from build123d import *

# Parameters (mm, degrees)
SKETCH_1_R          = 17.2
EXTRUDE_1_DEPTH     = 45
SKETCH_2_R          = 18.5
EXTRUDE_2_DEPTH     = 27
SKETCH_6_R          = 1.5
CUT_EXTRUDE_1_DEPTH = 10
SKETCH_3_R          = 6
EXTRUDE_3_DEPTH     = 8
SKETCH_4_R          = 3
EXTRUDE_4_DEPTH     = 15.5


with BuildPart() as part:
    # 草图1 → 凸台-拉伸1 (new body)
    with BuildSketch(Plane.XY):
        with Locations(Location((0, 0, 0), (0, 0, 180))):
            Circle(SKETCH_1_R)
    extrude(amount=EXTRUDE_1_DEPTH)

    # 草图2 → 凸台-拉伸2 (add)
    with BuildSketch(Plane.XY.offset(45)):
        Circle(SKETCH_2_R)
    extrude(amount=EXTRUDE_2_DEPTH)

    # 草图6 → 切除-拉伸1 (cut)
    with BuildSketch(Plane.XY.offset(72)):
        with Locations((-15.5, 0)):
            Circle(SKETCH_6_R)
        with Locations((-7.75, 13.423393759)):
            Circle(SKETCH_6_R)
        with Locations((7.75, 13.423393759)):
            Circle(SKETCH_6_R)
        with Locations((15.5, 0)):
            Circle(SKETCH_6_R)
        with Locations((7.75, -13.423393759)):
            Circle(SKETCH_6_R)
        with Locations((-7.75, -13.423393759)):
            Circle(SKETCH_6_R)
    extrude(amount=-CUT_EXTRUDE_1_DEPTH, mode=Mode.SUBTRACT)

    # 草图3 → 凸台-拉伸3 (add)
    with BuildSketch(Plane.XY.offset(72)):
        with Locations((0, 7)):
            Circle(SKETCH_3_R)
    extrude(amount=EXTRUDE_3_DEPTH)

    # 草图4 → 凸台-拉伸4 (add)
    with BuildSketch(Plane.XY.offset(80)):
        with Locations((0, 7)):
            Circle(SKETCH_4_R)
    extrude(amount=EXTRUDE_4_DEPTH)


solid = part.part
Part model, mm, in its own coordinate system. A direction names the side the tool comes from. Coordinates: 2 decimals unless noted, no trailing zeros. Loops run counter-clockwise (first coordinate to the right, second up) from the corner with the lowest first, then second, coordinate; pieces in that order, holes last. Notation, with made-up numbers: (39, -2.5) -> (56, -2.5) arc R12 cw to (56, 15.5) -> close; hole circle Ø9 at (4.5, 57.5). An arc over 180 degrees is marked (long way). Use a Markdown table: item, result. Add a question column.
Item 1: Probe probe 1 along Y at (x, z) = (-7.75, 67.25); probe 2 along Y at (x, z) = (7, 68); probe 3 along Z at (x, y) = (-7, -3). List the from-to ranges inside material, lowest first.
Item 2: Which spindle directions (+Z, -Z, +X, -X, +Y, -Y) get a long thin tool onto all of the face, cutting with end or side? Do faces 4 (the cylindrical face through (-17, 0, 67)), 5 (the flat face through (11, -14, 45)), 6 (the flat face through (0, 7, 95.5)). Say none if no direction does.
Item 3: Band-saw the part on A-A on y = 0. Write the cut outline in (x, z).
Item 4: Band-saw the part on D-D on y = 7. Write the cut outline in (x, z), plus the area to 3 significant figures.
Item 5: Flat gauge pins, fed straight in: P1, Ø3.5, axis at x = 15.5, y = -0.5, coming from the +Z side; P2, Ø1.5, axis at x = 8, y = -14, coming from the +Z side; P3, Ø10, axis at x = -3.5, y = -3, coming from the +Z side. Where does each tip first touch, or does it go through?
Item 6: Band-saw the part on C-C on z = 56. Write the cut outline in (x, y), plus the area to 3 significant figures.
Item 7: Pull direction Y, two halves, no side cores. Call faces 1 (the cylindrical face through (17.183, -0.756, 22.185)), 2 (the cylindrical face through (7.42, 11.96, 67.07)), 3 (the flat face through (1, 10, 80)): +Y half, -Y half, draft (parallel to the pull), parting line (faces both ways), or undercut.
Item 8: Band-saw the part on B-B on x = -15.5. Write the cut outline in (y, z).
Geometry says:
| question | item | result |
|---|---|---|
| 1 | probe 1 | -16.8 to -14.92, -11.92 to 11.92, 14.92 to 16.8 |
| 1 | probe 2 | -17.12 to -14.72, -12.12 to 12.12, 14.72 to 17.12 |
| 1 | probe 3 | 0 to 72 |
| 2 | face 4 | +Z |
| 2 | face 5 | -Z |
| 2 | face 6 | +Z, +X, -X, +Y, -Y |
| 3 | outline | (-18.5, 45) -> (-17.2, 45) -> (-17.2, 0) -> (17.2, 0) -> (17.2, 45) -> (18.5, 45) -> (18.5, 72) -> (17, 72) -> (17, 62) -> (14, 62) -> (14, 72) -> (-14, 72) -> (-14, 62) -> (-17, 62) -> (-17, 72) -> (-18.5, 72) -> close |
| 4 | outline | (-17.12, 45) -> (-15.71, 45) -> (-15.71, 0) -> (15.71, 0) -> (15.71, 45) -> (17.12, 45) -> (17.12, 72) -> (6, 72) -> (6, 80) -> (3, 80) -> (3, 95.5) -> (-3, 95.5) -> (-3, 80) -> (-6, 80) -> (-6, 72) -> (-17.12, 72) -> close |
| 4 | area | 2,530 mm² |
| 5 | P1 | z = 72 |
| 5 | P2 | z = 62 |
| 5 | P3 | z = 80 |
| 6 | outline | circle Ø37 at (0, 0) |
| 6 | area | 1,080 mm² |
| 7 | face 1 | parting line |
| 7 | face 2 | undercut |
| 7 | face 3 | draft |
| 8 | outline | (-10.1, 45) -> (-7.46, 45) -> (-7.46, 0) -> (7.46, 0) -> (7.46, 45) -> (10.1, 45) -> (10.1, 72) -> (1.5, 72) -> (1.5, 62) -> (-1.5, 62) -> (-1.5, 72) -> (-10.1, 72) -> close |
